Verification items for the finished model (mm, model axes). A direction names the side the tool comes from. Give positions to 0.01 mm unless a question says otherwise; leave off trailing zeros. Order: outer loops, then holes, each group sorted by start corner. A loop starts at its lowest first (then second) coordinate and runs counter-clockwise, first axis right, second up. Notation, with made-up numbers: (58.25, 78) -> (104.25, 78) arc R26 ccw to (104.25, 110) -> close; hole circle Ø6 at (-21.75, 30.25). An arc over 180 degrees is marked (long way). Return JSON: item names as keys, results as strings. Group by question number.
(1) Cross-section at B-B on y = 5.5. Enter the section's corners in (x, z), then the cut area to 3 significant figures.
(2) Tool access check on faces 1 (the face through (-1, 6, 37)), 2 (the face through (41.084, 5.542, 32.741)). Record the directions out of +Z, -Z, +X, -X, +Y, -Y that give a thin tool (end or side, any length) a straight path to the whole face; none if there is none.
(3) Release check for a two-part mould opening along X. For faces 3 (the face through (-1, 0, -1)), 4 (the face through (-42, 2.5, 33)), 5 (the face through (47, 6, 1)) record: pulls with the +X half, pulls with the -X half, needs draft (parallel to the pull), parting line crosses it, or undercut.
(4) Cross-section at A-A on x = 17.5. Enter the section's corners in (y, z).
(5) Thickness scan on line 1 along X through (y, z) = (0.9, 0); line 2 along Z through (x, y) = (38.5, 9); line 3 along X through (y, z) = (10.25, -16.5). Record the ranges inside material, lowest first.
(6) Depth check by flat-ended pin: pin 1 Ø3 at (x, z) = (27.5, -7.5) entering from +Y; pin 2 Ø2.5 at (x, z) = (-43, -32.5) entering from +Y; pin 3 Ø2.5 at (x, z) = (-42.5, -33.06) entering from +Y. Enter the tip coordinate at first touch or a pass-through.
(7) Cross-section at C-C on y = 10. Enter the section's corners in (x, z), then the cut area to 3 significant figures.
(8) Cross-section at D-D on z = -21. Enter the section's corners in (x, y).
from build123d import *

# Parameters (mm, degrees)
SKETCH1_W           = 94
SKETCH1_H           = 74
BOSS_EXTRUDE1_DEPTH = 12
SKETCH2_W           = 90.5
SKETCH2_H           = 70.5
CUT_EXTRUDE1_DEPTH  = 3.5
SKETCH3_R           = 1.45
CUT_EXTRUDE2_DEPTH  = 6
SHELL1_START        = 3
SHELL1_DEPTH        = 5.5
CHAMFER1_SIZE       = 1
CHAMFER2_SIZE       = 1
CHAMFER3_SIZE       = 1
SKETCH4_R           = 2.1
CUT_EXTRUDE3_DEPTH  = 61.489668539


# Read off the part's stored shape, not the designer's step: Shell1
with BuildPart() as part:
    # Sketch1 → Boss-Extrude1 (new body)
    with BuildSketch(Plane(origin=(0, 0, 0), x_dir=(1, 0, 0), z_dir=(0, 1, 0))):
        Rectangle(SKETCH1_W, SKETCH1_H)
    extrude(amount=BOSS_EXTRUDE1_DEPTH)

    # Sketch2 → Cut-Extrude1 (cut)
    with BuildSketch(Plane(origin=(0, 12, 0), x_dir=(1, 0, 0), z_dir=(0, 1, 0))):
        Rectangle(SKETCH2_W, SKETCH2_H)
    extrude(amount=-CUT_EXTRUDE1_DEPTH, mode=Mode.SUBTRACT)

    # Sketch3 → Cut-Extrude2 (cut)
    with BuildSketch(Plane(origin=(0, 8.5, 0), x_dir=(1, 0, 0), z_dir=(0, 1, 0))):
        with Locations(Location((-42.5, 33.055555556, 0), (0, 0, 270))):
            Circle(SKETCH3_R)
        with Locations(Location((42.5, 33.055555556, 0), (0, 0, 270))):
            Circle(SKETCH3_R)
        with Locations(Location((42.5, -33.055555556, 0), (0, 0, 270))):
            Circle(SKETCH3_R)
        with Locations(Location((-42.5, -33.055555556, 0), (0, 0, 270))):
            Circle(SKETCH3_R)
    extrude(amount=-CUT_EXTRUDE2_DEPTH, mode=Mode.SUBTRACT)

    # Shell1 outline → Shell1 (cut)
    with BuildSketch(Plane(origin=(0, 0, 0), x_dir=(1, 0, 0), z_dir=(0, 1, 0)).offset(SHELL1_START)):
        with BuildLine():
            Line((-38.15137669, -34), (38.15137669, -34))
            ThreePointArc((38.15137669, -34), (39.564324481, -29.711260526), (44, -28.865985172))
            Line((44, -28.865985172), (44, 28.865985172))
            ThreePointArc((44, 28.865985172), (39.564324481, 29.711260526), (38.15137669, 34))
            Line((38.15137669, 34), (-38.15137669, 34))
            ThreePointArc((-38.15137669, 34), (-39.564324481, 29.711260526), (-44, 28.865985172))
            Line((-44, 28.865985172), (-44, -28.865985172))
            ThreePointArc((-44, -28.865985172), (-39.564324481, -29.711260526), (-38.15137669, -34))
        make_face()
    extrude(amount=SHELL1_DEPTH, mode=Mode.SUBTRACT)

    # Chamfer1
    chamfer1_edges = [part.edges().sort_by_distance(p)[0] for p in [
        (45.25, 12, 0),
        (0, 12, -35.25),
        (-45.25, 12, 0),
        (0, 12, 35.25),
    ]]
    chamfer(chamfer1_edges, length=CHAMFER1_SIZE)

    # Chamfer2
    chamfer2_edges = [part.edges().sort_by_distance(p)[0] for p in [
        (0, 8.5, 34),
        (44, 8.5, 0),
        (0, 8.5, -34),
        (-44, 8.5, 0),
        (-39.564324481, 8.5, -29.711260526),
        (39.564324481, 8.5, -29.711260526),
        (39.564324481, 8.5, 29.711260526),
        (-39.564324481, 8.5, 29.711260526),
    ]]
    chamfer(chamfer2_edges, length=CHAMFER2_SIZE)

    # Chamfer3
    chamfer3_edges = [part.edges().sort_by_distance(p)[0] for p in [
        (-47, 6, 37),
        (-47, 6, -37),
        (47, 6, -37),
        (47, 6, 37),
    ]]
    chamfer(chamfer3_edges, length=CHAMFER3_SIZE)

    # Sketch4 → Cut-Extrude3 (cut, through all)
    with BuildSketch(Plane(origin=(0, 3, 0), x_dir=(1, 0, 0), z_dir=(0, 1, 0))):
        with Locations(Location((-17.5, 0, 0), (0, 0, 270))):
            Circle(SKETCH4_R)
        with Locations(Location((17.5, 0, 0), (0, 0, 270))):
            Circle(SKETCH4_R)
    extrude(amount=-CUT_EXTRUDE3_DEPTH, mode=Mode.SUBTRACT)


solid = part.part
Verdict:
{
 "1": {"outline": "(-47, -36) -> (-46, -37) -> (46, -37) -> (47, -36) -> (47, 36) -> (46, 37) -> (-46, 37) -> (-47, 36) -> close; hole (-44, -28.87) arc R4.45 cw to (-38.15, -34) -> (38.15, -34) arc R4.45 cw to (44, -28.87) -> (44, 28.87) arc R4.45 cw to (38.15, 34) -> (-38.15, 34) arc R4.45 cw to (-44, 28.87) -> close; hole circle Ø2.9 at (-42.5, -33.06); hole circle Ø2.9 at (-42.5, 33.06); hole circle Ø2.9 at (42.5, -33.06); hole circle Ø2.9 at (42.5, 33.06)", "area": "1,050 mm²"},
 "2": {"face 1": "+Z, +X, -X, +Y, -Y", "face 2": "+Y"},
 "3": {"face 3": "needs draft", "face 4": "undercut", "face 5": "pulls with the +X half"},
 "4": {"outline": "(0, -37) -> (12, -37) -> (12, -36.25) -> (11, -35.25) -> (8.5, -35.25) -> (8.5, -35) -> (7.5, -34) -> (3, -34) -> (3, -2.1) -> (0, -2.1) -> close; (0, 2.1) -> (3, 2.1) -> (3, 34) -> (7.5, 34) -> (8.5, 35) -> (8.5, 35.25) -> (11, 35.25) -> (12, 36.25) -> (12, 37) -> (0, 37) -> close"},
 "5": {"line 1": "-47 to -19.6, -15.4 to 15.4, 19.6 to 47", "line 2": "-37 to -35.25, 35.25 to 37", "line 3": "-47 to -45.25, 45.25 to 47"},
 "6": {"pin 1": "y = 3", "pin 2": "y = 8.5", "pin 3": "y = 2.5"},
 "7": {"outline": "(-47, -36) -> (-46, -37) -> (46, -37) -> (47, -36) -> (47, 36) -> (46, 37) -> (-46, 37) -> (-47, 36) -> close; hole (-45.25, -35.25) -> (45.25, -35.25) -> (45.25, 35.25) -> (-45.25, 35.25) -> close", "area": "574 mm²"},
 "8": {"outline": "(-47, 0) -> (47, 0) -> (47, 12) -> (46.25, 12) -> (45.25, 11) -> (45.25, 8.5) -> (45, 8.5) -> (44, 7.5) -> (44, 3) -> (-44, 3) -> (-44, 7.5) -> (-45, 8.5) -> (-45.25, 8.5) -> (-45.25, 11) -> (-46.25, 12) -> (-47, 12) -> close"}
}
